```python
from build123d import *

# Parameters (mm, degrees)
SKETCH1_W           = 100
SKETCH1_H           = 8
BOSS_EXTRUDE1_DEPTH = 35
SKETCH2_W           = 100
SKETCH2_H           = 8
BOSS_EXTRUDE2_DEPTH = 40
SKETCH6_W           = 60
SKETCH6_H           = 8
CUT_EXTRUDE2_DEPTH  = 10
FILLET1_R           = 10
SKETCH8_W           = 100
SKETCH8_H           = 8
BOSS_EXTRUDE3_DEPTH = 35
CUT_EXTRUDE3_DEPTH  = 8
FILLET2_R           = 5


with BuildPart() as part:
    # Sketch1 → Boss-Extrude1 (new body)
    with BuildSketch(Plane(origin=(0, 0, 0), x_dir=(1, 0, 0), z_dir=(0, 1, 0))):
        with Locations((-50, -4)):
            Rectangle(SKETCH1_W, SKETCH1_H)
    extrude(amount=BOSS_EXTRUDE1_DEPTH)

    # Sketch2 → Boss-Extrude2 (add)
    with BuildSketch(Plane.XY):
        with Locations((-50, 31)):
            Rectangle(SKETCH2_W, SKETCH2_H)
    extrude(amount=BOSS_EXTRUDE2_DEPTH)

    # Sketch6 → Cut-Extrude2 (cut)
    with BuildSketch(Plane.XY.offset(40)):
        with Locations((-50, 31)):
            Rectangle(SKETCH6_W, SKETCH6_H)
    extrude(amount=-CUT_EXTRUDE2_DEPTH, mode=Mode.SUBTRACT)

    # Fillet1
    fillet1_edges = [part.edges().sort_by_distance(p)[0] for p in [
        (-20, 31, 30),
        (-80, 31, 30),
    ]]
    fillet(fillet1_edges, radius=FILLET1_R - 0.0001)  # a hair under: the kernel refuses the full size

    # Sketch8 → Boss-Extrude3 (add)
    with BuildSketch(Plane(origin=(0, 35, 0), x_dir=(1, 0, 0), z_dir=(0, 1, 0))):
        with Locations((-50, -15)):
            Rectangle(SKETCH8_W, SKETCH8_H)
    extrude(amount=BOSS_EXTRUDE3_DEPTH)

    # Sketch9 → Cut-Extrude3 (cut)
    with BuildSketch(Plane.XY.offset(19)):
        with BuildLine():
            Line((-85, 70), (-85, 56))
            ThreePointArc((-85, 56), (-80, 51), (-75, 56))
            Line((-75, 56), (-75, 70))
            Line((-75, 70), (-85, 70))
        make_face()
        with BuildLine():
            Line((-65, 70), (-65, 56))
            ThreePointArc((-65, 56), (-60, 51), (-55, 56))
            Line((-55, 56), (-55, 70))
            Line((-55, 70), (-65, 70))
        make_face()
        with BuildLine():
            Line((-45, 70), (-45, 56))
            ThreePointArc((-45, 56), (-40, 51), (-35, 56))
            Line((-35, 56), (-35, 70))
            Line((-35, 70), (-45, 70))
        make_face()
        with BuildLine():
            Line((-25, 70), (-25, 56))
            ThreePointArc((-25, 56), (-20, 51), (-15, 56))
            Line((-15, 56), (-15, 70))
            Line((-15, 70), (-25, 70))
        make_face()
    extrude(amount=-CUT_EXTRUDE3_DEPTH, mode=Mode.SUBTRACT)

    # Fillet2
    fillet2_edges = [part.edges().sort_by_distance(p)[0] for p in [
        (-50, 35, 19),
    ]]
    fillet(fillet2_edges, radius=FILLET2_R)


solid = part.part
```
The listing builds one solid part. Answer for the finished solid, in the listing's coordinates (mm). A direction names the side the tool comes from. Coordinates: 2 decimals unless noted, no trailing zeros. Write each loop counter-clockwise with the first axis right and the second up, starting at its lowest first coordinate (ties: lowest second). Pieces come first, ordered by that corner, then holes. Notation, with made-up numbers: (57.5, 41.5) - (116.5, 41.5) arc R20 cw to (116.5, 75.5) - close; hole circle Ø4 at (40.25, 64). An arc over 180 degrees is marked (long way). One line per item, written item: value.
1) Find section A-A (x = -10). Give the vertices of the cut face in (y, z).
Geometry check:
outline: (0, 0) - (35, 0) - (35, 11) - (70, 11) - (70, 19) - (40, 19) arc R5 cw to (35, 24) - (35, 40) - (27, 40) - (27, 8) - (0, 8) - close
2) Find section C-C (y = 54). Give the vertices of the cut face in (x, z), and give its area (3 significant figures).
Geometry check:
outline: (-100, 11) - (-84.58, 11) - (-84.58, 19) - (-100, 19) - close; (-75.42, 11) - (-64.58, 11) - (-64.58, 19) - (-75.42, 19) - close; (-55.42, 11) - (-44.58, 11) - (-44.58, 19) - (-55.42, 19) - close; (-35.42, 11) - (-24.58, 11) - (-24.58, 19) - (-35.42, 19) - close; (-15.42, 11) - (0, 11) - (0, 19) - (-15.42, 19) - close
area: 507 mm2
3) Find section B-B (z = 15). Give the vertices of the cut face in (x, y).
Geometry check:
outline: (-100, 27) - (0, 27) - (0, 70) - (-15, 70) - (-15, 56) arc R5 cw to (-25, 56) - (-25, 70) - (-35, 70) - (-35, 56) arc R5 cw to (-45, 56) - (-45, 70) - (-55, 70) - (-55, 56) arc R5 cw to (-65, 56) - (-65, 70) - (-75, 70) - (-75, 56) arc R5 cw to (-85, 56) - (-85, 70) - (-100, 70) - close
4) For a pull along X with two mould halves and no side action, classify faces 1 (the flat face through (-51, 27, 20)), 2 (the flat face through (0, 32, 14)), 3 (the flat face through (-55, 63, 15)) as pulls with the +X half, pulls with the -X half, needs draft (parallel to the pull), parting line crosses it, or undercut.
Geometry check:
face 1: needs draft
face 2: pulls with the +X half
face 3: undercut
5) Each of these flat-tipped pins is pushed along its axis until it touches: pin 1 Ø5 at (x, y) = (-56, 21.5) entering from +Z; pin 2 Ø1 at (x, z) = (-15.5, 31) entering from -Y; pin 3 Ø5.5 at (x, z) = (-74.5, 4.5) entering from +Y. Where does it stop, or does it pass through?
Geometry check:
pin 1: stops at z = 8
pin 2: stops at y = 27
pin 3: stops at y = 35
6) Consider line 1 along Z through (x, y) = (-5.5, 61); line 2 along Y through (x, z) = (-30.5, 7); line 3 along Y through (x, z) = (-83, 26.5). Determine where each line is inside the solid, lowest interval first. Write a range as from..to.
Geometry check:
line 1: z = 11..19
line 2: y = 0..35
line 3: y = 27..35
7) A tool of negligible diameter and unlimited length cuts with its end or side. For faces 4 (the flat face through (-85, 63, 15)), 5 (the flat face through (-51, 35, 28)), 6 (the flat face through (-51, 48, 11)), 7 (the flat face through (-50, 31, 30)), from which of +Z, -Z, +X, -X, +Y, -Y can it reach the whole face along a straight path? Write none if from no direction.
Geometry check:
face 4: +Z, -Z, +Y
face 5: +Z, +X, -X, +Y
face 6: -Z, +X, -X, +Y
face 7: +Z, +Y, -Y
